The model under review builds one solid part; all positions refer to its coordinate system, in mm. A direction names the side the tool comes from. Coordinates: 2 decimals unless noted, no trailing zeros. Order: outer loops, then holes, each group sorted by start corner. A loop starts at its lowest first (then second) coordinate and runs counter-clockwise, first axis right, second up.
```python
from build123d import *

# Parameters (mm, degrees)
F0_W     = 812
F0_H     = 1306
F0_W_2   = 712
F0_H_2   = 1206
F1_DEPTH = 1
F2_W     = 808
F2_H     = 1302
F2_W_2   = 804
F2_H_2   = 1298
F2_W_3   = 716
F2_H_3   = 1210
F2_W_4   = 712
F2_H_4   = 1206
F3_DEPTH = 36
F4_W     = 836
F4_H     = 1330
F4_W_2   = 712
F4_H_2   = 1206
F5_DEPTH = 2


with BuildPart() as f1:
    # F0 (on Front) → F1 (new body, symmetric)
    with BuildSketch(Plane.XZ):
        Rectangle(F0_W, F0_H)
        Rectangle(F0_W_2, F0_H_2, mode=Mode.SUBTRACT)
    extrude(amount=F1_DEPTH, both=True)

    # F2 (on face) → F3 (join)
    with BuildSketch(Plane.XZ.offset(1)):
        Rectangle(F2_W, F2_H)
        Rectangle(F2_W_2, F2_H_2, mode=Mode.SUBTRACT)
        Rectangle(F2_W_3, F2_H_3)
        Rectangle(F2_W_4, F2_H_4, mode=Mode.SUBTRACT)
    extrude(amount=F3_DEPTH)

    # F4 (on face) → F5 (join)
    with BuildSketch(Plane.XZ.offset(37)):
        Rectangle(F4_W, F4_H)
        Rectangle(F4_W_2, F4_H_2, mode=Mode.SUBTRACT)
    extrude(amount=F5_DEPTH)


solid = f1.part
```
(1) We need section C-C, the plane y = -27. Write out the cut boundary in (x, z), and give its area (3 significant figures).
A:
outline: (-404, -651) - (404, -651) - (404, 651) - (-404, 651) - close; (-358, -605) - (358, -605) - (358, 605) - (-358, 605) - close; hole (-402, -649) - (402, -649) - (402, 649) - (-402, 649) - close; hole (-356, -603) - (356, -603) - (356, 603) - (-356, 603) - close
area: 16,100 mm2
(2) We need section B-B, the plane z = 355.5. Write out the cut boundary in (x, y).
A:
outline: (-418, -39) - (-356, -39) - (-356, 1) - (-406, 1) - (-406, -1) - (-404, -1) - (-404, -37) - (-418, -37) - close; (356, -39) - (418, -39) - (418, -37) - (404, -37) - (404, -1) - (406, -1) - (406, 1) - (356, 1) - close; hole (-402, -37) - (-358, -37) - (-358, -1) - (-402, -1) - close; hole (358, -37) - (402, -37) - (402, -1) - (358, -1) - close
(3) Machinability: for faces 4 (the face through (-363, 1, 51)), 5 (the face through (-5, -19, 603)), 6 (the face through (-5, -19, -605)), 7 (the face through (-404, -19, -9)), which of the approach directions +Z, -Z, +X, -X, +Y, -Y give a long, thin tool a straight path to every point of the face, cutting with its end or side? Answer none if there is none.
A:
face 4: +Z, -Z, +X, -X, +Y
face 5: +Y, -Y
face 6: none
face 7: +Z, -Z, -X
(4) Wall thickness on probe 1 along Z at (x, y) = (-264, -30.5); probe 2 along X at (y, z) = (-1.5, -394.5); probe 3 along Z at (x, y) = (-365, -24.5): over which ranges is each line inside the solid? List them lowest first.
A:
probe 1: z = -651 to -649, -605 to -603, 603 to 605, 649 to 651
probe 2: x = -404 to -402, -358 to -356, 356 to 358, 402 to 404
probe 3: z = -651 to -649, 649 to 651
(5) Draft analysis for pull direction X (two halves, no side actions). For faces 1 (the face through (-6, -19, 651)), 2 (the face through (-359, -1, 3)), 3 (the face through (404, -19, -9)), state which applies: released by +X, released by -X, zero draft, split by the parting line, or undercut.
A:
face 1: zero draft
face 2: undercut
face 3: released by +X
(6) For pin 1 Ø8 at (x, y) = (120.5, -31.5) entering from +Z; pin 2 Ø11 at (y, z) = (-19, -187) entering from -X; pin 3 Ø6 at (y, z) = (-28, 368) entering from +X, all flat-tipped, find the tip position at first contact; note any pin that passes through.
A:
pin 1: stops at z = 651
pin 2: stops at x = -404
pin 3: stops at x = 404
(7) We need section A-A, the plane x = 229. Write out the cut boundary in (y, z), and give its area (3 significant figures).
A:
outline: (-39, -665) - (-37, -665) - (-37, -651) - (-1, -651) - (-1, -653) - (1, -653) - (1, -603) - (-39, -603) - close; (-39, 603) - (1, 603) - (1, 653) - (-1, 653) - (-1, 651) - (-37, 651) - (-37, 665) - (-39, 665) - close; hole (-37, -649) - (-1, -649) - (-1, -605) - (-37, -605) - close; hole (-37, 605) - (-1, 605) - (-1, 649) - (-37, 649) - close
area: 736 mm2
